```python
from build123d import *

# Parameters (mm, degrees)
BASE_SKETCH_W          = 9.4
BASE_SKETCH_H          = 18.5
BASE_DEPTH             = 5
BASE_TOP_DEPTH         = 5
MAN_OP_CUTOUT_SKETCH_R = 1.7
MAN_OP_CUTOUT_DEPTH    = 0.5


with BuildPart() as part:
    # Base Sketch → Base (new, symmetric)
    with BuildSketch(Plane.XY):
        with Locations((-4.7, 9.25)):
            Rectangle(BASE_SKETCH_W, BASE_SKETCH_H)
    extrude(amount=BASE_DEPTH, both=True)

    # Base Top Sketch → Base Top (add, symmetric)
    with BuildSketch(Plane.XY):
        Polygon((-2.758330249, 18.5), (-9.4, 18.5), (-9.4, 25), (-4.5, 25), align=None)
    extrude(amount=BASE_TOP_DEPTH, both=True)

    # Man-op cutout sketch → Man-op cutout (cut)
    with BuildSketch(Plane(origin=(0, 25, 0), x_dir=(-1, 0, 0), z_dir=(0, 1, 0))):
        with Locations(Location((6.7, 0, 0), (0, 0, 90))):
            Circle(MAN_OP_CUTOUT_SKETCH_R)
    extrude(amount=-MAN_OP_CUTOUT_DEPTH, mode=Mode.SUBTRACT)


solid = part.part
```
The listing builds one solid part. Answer for the finished solid, in the listing's coordinates (mm). A direction names the side the tool comes from. Coordinates: 2 decimals unless noted, no trailing zeros. Loops run counter-clockwise (first coordinate to the right, second up) from the corner with the lowest first, then second, coordinate; pieces in that order, holes last. Notation, with made-up numbers: (0.5, -7.75) -> (36.5, -7.75) arc R32 cw to (36.5, 30.25) -> close; hole circle Ø7 at (35, 57). An arc over 180 degrees is marked (long way). Use one line per item in the form item = value. Start each with the question number.
Item 1: A tool of negligible diameter and unlimited length cuts with its end or side. For faces 4 (the face through (-9.4, 12, 0)), 5 (the face through (-1, 18.5, 0)), 6 (the face through (-7, 24.5, 0)), from which of +Z, -Z, +X, -X, +Y, -Y can it reach the whole face along a straight path? Write none if from no direction.
Item 2: The part is cut by section A-A on z = 2.5. Determine the outline of the cut face in (x, y).
Item 3: The part is cut by section B-B on x = -3. Determine the outline of the cut face in (y, z).
Item 4: Consider L1, parallel to Y at x = -2, z = -2; L2, parallel to X at y = 24.8, z = 0; L3, parallel to X at y = 24.95, z = 0. Determine where each line is inside the solid, lowest interval first. Write a range as [from, to].
Item 5: The mould has two halves that part along Z. Classify faces 1 (the face through (-5, 13, 5)), 2 (the face through (0, 9, 0)), 3 (the face through (-5.267, 24.754, 0.914)): released by +Z, released by -Z, zero draft, split by the parting line, or undercut.
Item 6: The part is cut by section D-D on y = 23. Determine the outline of the cut face in (x, z).
Item 7: Flat-ended cylindrical pins translate along their axes: pin 1 Ø0.8 at (x, z) = (-1, 1) entering from +Y; pin 2 Ø3 at (x, z) = (-6.7, 0) entering from +Y. Find the tip coordinate at first contact, or state that the pin passes through.
Item 8: The part is cut by section C-C on z = 0.5. Determine the outline of the cut face in (x, y), then the cut area to 3 significant figures.
Answer key:
q1.face_4 = +Z, -Z, -X, +Y, -Y
q1.face_5 = +Z, -Z, +X, +Y
q1.face_6 = +Y
q2.outline = (-9.4, 0) -> (0, 0) -> (0, 18.5) -> (-2.76, 18.5) -> (-4.5, 25) -> (-9.4, 25) -> close
q3.outline = (0, -5) -> (19.4, -5) -> (19.4, 5) -> (0, 5) -> close
q4.L1 = [0, 18.5]
q4.L2 = [-9.4, -8.4], [-5, -4.45]
q4.L3 = [-9.4, -8.4], [-5, -4.49]
q5.face_1 = released by +Z
q5.face_2 = zero draft
q5.face_3 = undercut
q6.outline = (-9.4, -5) -> (-3.96, -5) -> (-3.96, 5) -> (-9.4, 5) -> close
q7.pin_1 = 18.5
q7.pin_2 = 24.5
q8.outline = (-9.4, 0) -> (0, 0) -> (0, 18.5) -> (-2.76, 18.5) -> (-4.5, 25) -> (-5.08, 25) -> (-5.08, 24.5) -> (-8.32, 24.5) -> (-8.32, 25) -> (-9.4, 25) -> close
q8.area = 210 mm2
